The drawing under review shows one solid part. Ordinate dimensions are in mm from its lowest x, y, z. Coordinates: 2 decimals unless noted, no trailing zeros. Order: outer loops, then holes, each group sorted by start corner. A loop starts at its lowest first (then second) coordinate and runs counter-clockwise, first axis right, second up. Notation, with made-up numbers: (73, 63.25) -> (77, 63.25) arc R38 ccw to (77, 102.25) -> close; hole circle Ø8 at (59, -32.75). An arc over 180 degrees is marked (long way). Put each result on its own line as item: value.
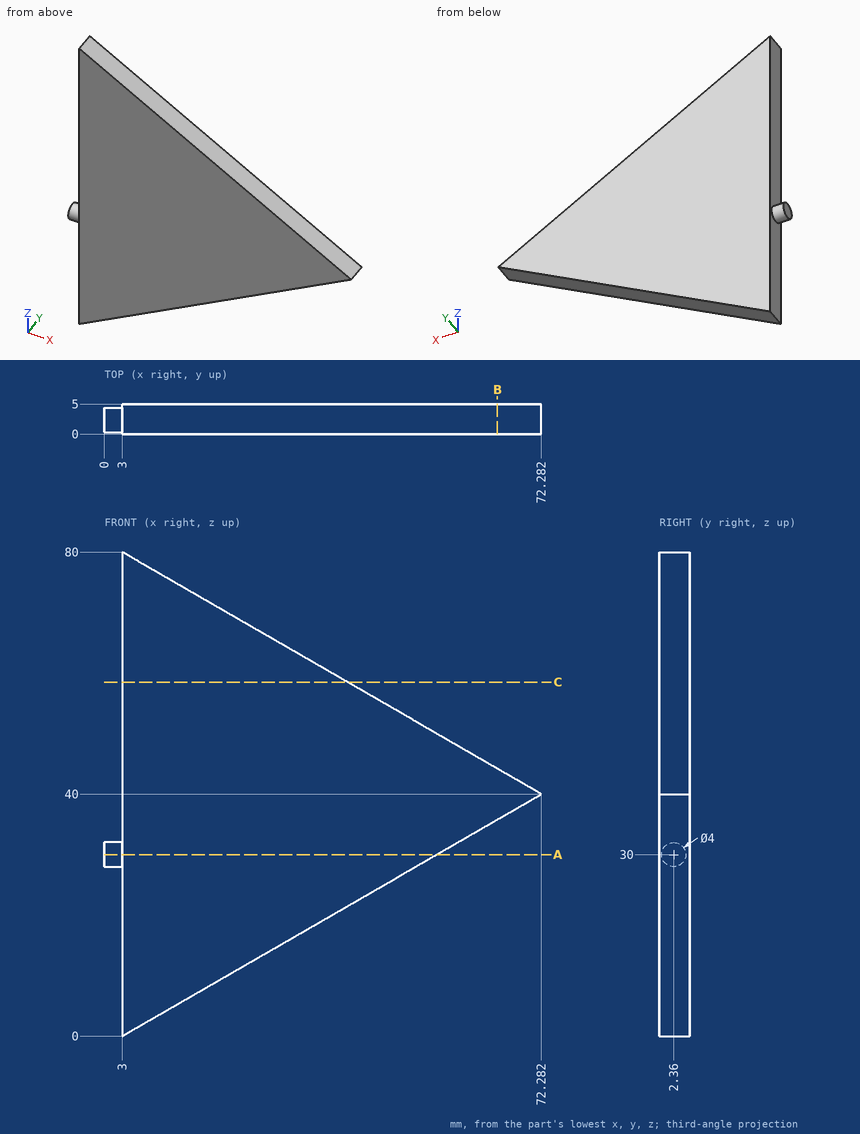
Item 1: Consider section A-A on z = 30. Write out the cut boundary in (x, y), and give its area (3 significant figures).
Answers below:
outline: (0, 0.36) -> (3, 0.36) -> (3, 0) -> (54.96, 0) -> (54.96, 5) -> (3, 5) -> (3, 4.36) -> (0, 4.36) -> close
area: 272 mm^2
Item 2: Consider section C-C on z = 58.5. Write out the cut boundary in (x, y), and give its area (3 significant figures).
Answers below:
outline: (3, 0) -> (40.24, 0) -> (40.24, 5) -> (3, 5) -> close
area: 186 mm^2
Item 3: Consider section B-B on x = 65. Write out the cut boundary in (y, z).
Answers below:
outline: (0, 35.8) -> (5, 35.8) -> (5, 44.2) -> (0, 44.2) -> close
Item 4: For line 1 (Z direction, x = 36.5, y = 4.7); line 2 (Z direction, x = 55.5, y = 2.4); line 3 (X direction, y = 4.65, z = 28), list the stretches that pass through material, from the lowest coordinate up. Write a range as from..to.
Answers below:
line 1: 19.34..60.66
line 2: 30.31..49.69
line 3: 3..51.5
Item 5: For pin 1 Ø1.5 at (x, y) = (55, 2.5) entering from -Z; pin 2 Ø3 at (y, z) = (2.5, 61) entering from +X, all flat-tipped, find the tip position at first contact; note any pin that passes through.
Answers below:
pin 1: z = 29.59
pin 2: x = 38.51
